CAD build for the part. Positions are in the model's coordinates, mm. A direction names the side the tool comes from. Coordinates: 2 decimals unless noted, no trailing zeros. Write each loop counter-clockwise with the first axis right and the second up, starting at its lowest first coordinate (ties: lowest second). Pieces come first, ordered by that corner, then holes. Notation, with made-up numbers: (65.5, 22.5) - (69.5, 22.5) arc R11 cw to (69.5, 38.5) - close; hole circle Ø5 at (44, 26.5). An arc over 180 degrees is marked (long way). One line per question, with ' | ' between items. Start each with the question number.
1. Flat gauge pins, fed straight in: P1, Ø10, axis at x = 39.5, z = 5, coming from the +Y side; P2, Ø2.5, axis at x = 58, z = 6, coming from the +Y side; P3, Ø3.5, axis at y = 6.5, z = 5, coming from the -X side. Where does each tip first touch, or does it go through?
2. Band-saw the part on D-D, the plane y = 6. Write the cut outline in (x, z).
3. Two-plate mould, pull along X, no slides. Class faces 4 (the cylindrical face through (59.55, 3.84, -5.36)), 5 (the flat face through (43, 3, 5)), 6 (the flat face through (25.481, 3, 5)), 7 (the flat face through (27, 6, 9.066)): +X half, -X half, draft (parallel to the pull), parting line (faces both ways), or undercut.
4. Which spindle directions (+Z, -Z, +X, -X, +Y, -Y) get a long thin tool onto all of the face, cutting with end or side? Do faces 1 (the flat face through (27, 4.006, 5)), 2 (the flat face through (28, 1.382, 13)), 3 (the flat face through (58, 6.464, 5)). Say none if no direction does.
5. Band-saw the part on A-A, the plane x = 31. Write the cut outline in (y, z), then the cut area to 3 significant figures.
6. Probe line 1 (X direction, y = 4, z = 10.25); line 2 (Z direction, x = 51, y = 5.5); line 3 (X direction, y = 4.25, z = 12.5) (3 decimals). List the from-to ranges inside material, lowest first.
7. Band-saw the part on C-C, the plane y = 2. Write the cut outline in (x, z).
8. Band-saw the part on B-B, the plane z = 6.5. Write the cut outline in (x, y), then the cut area to 3 significant figures.
from build123d import *

# Parameters (mm, degrees)
SKETCH1_W           = 34.447999938
SKETCH1_H           = 20.985999938
BOSS_EXTRUDE1_DEPTH = 7.572
SKETCH3_W           = 28.448
SKETCH3_H           = 14.986
CUT_EXTRUDE1_DEPTH  = 4.572
SKETCH4_R           = 1
CUT_EXTRUDE2_DEPTH  = 6.19
FILLET1_R           = 1.27
FILLET2_R           = 0.254
FILLET3_R           = 0.254
SKETCH5_W           = 8.599089175
SKETCH5_H           = 3.565628699
CUT_EXTRUDE3_DEPTH  = 2.999999969
FILLET4_R           = 0.508
SKETCH7_W           = 7.982788435
SKETCH7_H           = 1.108191991
CUT_EXTRUDE4_DEPTH  = 2.999999969
FILLET5_R           = 0.762


with BuildPart() as part:
    # Sketch1 → Boss-Extrude1 (new body)
    with BuildSketch(Plane(origin=(0, 0, 0), x_dir=(1, 0, 0), z_dir=(0, 1, 0))):
        with Locations((42.705323942, -4.766172171)):
            Rectangle(SKETCH1_W, SKETCH1_H)
    extrude(amount=BOSS_EXTRUDE1_DEPTH)

    # Sketch3 → Cut-Extrude1 (cut)
    with BuildSketch(Plane(origin=(0, 7.572, 0), x_dir=(1, 0, 0), z_dir=(0, 1, 0))):
        with Locations((42.705323942, -4.766172171)):
            Rectangle(SKETCH3_W, SKETCH3_H)
    extrude(amount=-CUT_EXTRUDE1_DEPTH, mode=Mode.SUBTRACT)

    # Sketch4 → Cut-Extrude2 (cut)
    with BuildSketch(Plane(origin=(0, 7.572, 0), x_dir=(1, 0, 0), z_dir=(0, 1, 0))):
        with Locations(Location((57.677427469, 3.474931356, 0), (0, 0, 270))):
            Circle(SKETCH4_R)
        with Locations(Location((57.677427469, -13.007275697, 0), (0, 0, 270))):
            Circle(SKETCH4_R)
        with Locations(Location((27.733220415, -13.007275697, 0), (0, 0, 270))):
            Circle(SKETCH4_R)
        with Locations(Location((27.733220415, 3.474931356, 0), (0, 0, 270))):
            Circle(SKETCH4_R)
    extrude(amount=-CUT_EXTRUDE2_DEPTH, mode=Mode.SUBTRACT)

    # Fillet1
    fillet1_edges = [part.edges().sort_by_distance(p)[0] for p in [
        (25.481323973, 3.786, -5.726827798),
        (59.929323911, 3.786, -5.726827798),
        (59.929323911, 3.786, 15.25917214),
        (25.481323973, 3.786, 15.25917214),
    ]]
    fillet(fillet1_edges, radius=FILLET1_R)

    # Fillet2
    fillet2_edges = [part.edges().sort_by_distance(p)[0] for p in [
        (28.481323942, 5.286, 12.259172171),
        (28.481323942, 5.286, -2.726827829),
        (56.929323942, 5.286, -2.726827829),
        (56.929323942, 5.286, 12.259172171),
    ]]
    fillet(fillet2_edges, radius=FILLET2_R)

    # Fillet3
    fillet3_edges = [part.edges().sort_by_distance(p)[0] for p in [
        (42.705323942, 3, -2.726827829),
        (56.929323942, 3, 4.766172171),
        (28.481323942, 3, 4.766172171),
        (42.705323942, 3, 12.259172171),
        (28.555718819, 3, -2.652432952),
        (28.555718819, 3, 12.184777293),
        (56.854929064, 3, 12.184777293),
        (56.854929064, 3, -2.652432952),
    ]]
    fillet(fillet3_edges, radius=FILLET3_R)

    # Sketch5 → Cut-Extrude3 (cut)
    with BuildSketch(Plane.ZY.offset(-25.481323973)):
        with Locations((4.76617217, 5.789185651)):
            Rectangle(SKETCH5_W, SKETCH5_H)
    extrude(amount=-CUT_EXTRUDE3_DEPTH, mode=Mode.SUBTRACT)

    # Fillet4
    fillet4_edges = [part.edges().sort_by_distance(p)[0] for p in [
        (26.981323957, 4.006371301, 9.065716758),
        (26.981323957, 4.006371301, 0.466627583),
    ]]
    fillet(fillet4_edges, radius=FILLET4_R)

    # Sketch7 → Cut-Extrude4 (cut)
    with BuildSketch(Plane(origin=(59.929323911, 0, 0), x_dir=(0, 0, -1), z_dir=(1, 0, 0))):
        with Locations((-4.766172171, 7.017904005)):
            Rectangle(SKETCH7_W, SKETCH7_H)
    extrude(amount=-CUT_EXTRUDE4_DEPTH, mode=Mode.SUBTRACT)

    # Fillet5
    fillet5_edges = [part.edges().sort_by_distance(p)[0] for p in [
        (58.429323926, 6.463808009, 0.774777953),
        (58.429323926, 6.463808009, 8.757566388),
    ]]
    fillet(fillet5_edges, radius=FILLET5_R)


solid = part.part
Filled in:
1) P1: stops at y = 3 | P2: stops at y = 6.46 | P3: stops at x = 56.93
2) outline: (25.48, -4.46) arc R1.27 ccw to (26.75, -5.73) - (58.66, -5.73) arc R1.27 ccw to (59.93, -4.46) - (59.93, 13.99) arc R1.27 ccw to (58.66, 15.26) - (26.75, 15.26) arc R1.27 ccw to (25.48, 13.99) - (25.48, 9.07) - (28.48, 9.07) - (28.48, 12.01) arc R0.25 cw to (28.74, 12.26) - (56.68, 12.26) arc R0.25 cw to (56.93, 12.01) - (56.93, -2.47) arc R0.25 cw to (56.68, -2.73) - (28.74, -2.73) arc R0.25 cw to (28.48, -2.47) - (28.48, 0.47) - (25.48, 0.47) - close; hole circle Ø2 at (27.73, -3.47); hole circle Ø2 at (27.73, 13.01); hole circle Ø2 at (57.68, -3.47); hole circle Ø2 at (57.68, 13.01)
3) face 4: +X half | face 5: undercut | face 6: -X half | face 7: draft
4) face 1: -X, +Y | face 2: +Y | face 3: +X, -X, +Y
5) outline: (0, -5.73) - (7.57, -5.73) - (7.57, -2.73) - (3.25, -2.73) arc R0.25 cw to (3, -2.47) - (3, 12.01) arc R0.25 cw to (3.25, 12.26) - (7.57, 12.26) - (7.57, 15.26) - (0, 15.26) - close | area: 90.4 mm²
6) line 1: x = 25.48 to 28.48, 56.93 to 59.93 | line 2: z = -5.73 to -2.73, 12.26 to 15.26 | line 3: x = 25.481 to 26.871, 28.595 to 56.816, 58.539 to 59.929
7) outline: (25.48, -4.46) arc R1.27 ccw to (26.75, -5.73) - (58.66, -5.73) arc R1.27 ccw to (59.93, -4.46) - (59.93, 13.99) arc R1.27 ccw to (58.66, 15.26) - (26.75, 15.26) arc R1.27 ccw to (25.48, 13.99) - close; hole circle Ø2 at (27.73, -3.47); hole circle Ø2 at (27.73, 13.01); hole circle Ø2 at (57.68, -3.47); hole circle Ø2 at (57.68, 13.01)
8) outline: (25.48, 0) - (59.93, 0) - (59.93, 6.46) - (56.93, 6.46) - (56.93, 3.25) arc R0.25 cw to (56.68, 3) - (28.74, 3) arc R0.25 cw to (28.48, 3.25) - (28.48, 4.01) - (25.48, 4.01) - close | area: 117 mm²
